The model under review builds one solid part; all positions refer to its coordinate system, in mm. A direction names the side the tool comes from. Give positions to 0.01 mm unless a question says otherwise; leave off trailing zeros. Loops run counter-clockwise (first coordinate to the right, second up) from the corner with the lowest first, then second, coordinate; pieces in that order, holes last. Notation, with made-up numbers: (1.25, -30.5) - (47.25, -30.5) arc R15 cw to (47.25, -11.5) - close; hole circle Ø3 at (-24, 44.25). An arc over 180 degrees is marked (long way). Answer as a JSON object with one key per item and string values.
from build123d import *

# Parameters (mm, degrees)
CROQUIS1_R              = 57
CROQUIS1_R_2            = 55.5
SALIENTE_EXTRUIR1_DEPTH = 530
CROQUIS2_R              = 10.65
CORTAR_EXTRUIR1_DEPTH   = 10
CROQUIS3_R              = 10.65
CORTAR_EXTRUIR3_DEPTH   = 10
CROQUIS4_W              = 120
CROQUIS4_H              = 120
CORTAR_EXTRUIR4_DEPTH   = 36
CORTAR_EXTRUIR5_DEPTH   = 36


with BuildPart() as part:
    # Croquis1 → Saliente-Extruir1 (new body)
    with BuildSketch(Plane(origin=(0, 0, 0), x_dir=(1, 0, 0), z_dir=(0, 1, 0))):
        with Locations(Location((0, 0, 0), (0, 0, 270))):
            Circle(CROQUIS1_R)
        with Locations(Location((0, 0, 0), (0, 0, 270))):
            Circle(CROQUIS1_R_2, mode=Mode.SUBTRACT)
    extrude(amount=SALIENTE_EXTRUIR1_DEPTH)

    # Croquis2 → Cortar-Extruir1 (cut)
    with BuildSketch(Plane.ZY.offset(57)):
        with Locations((0, 440)):
            Circle(CROQUIS2_R)
    extrude(amount=-CORTAR_EXTRUIR1_DEPTH, mode=Mode.SUBTRACT)

    # Croquis3 → Cortar-Extruir3 (cut)
    with BuildSketch(Plane(origin=(57, 0, 0), x_dir=(0, 0, -1), z_dir=(1, 0, 0))):
        with Locations((0, 38.1)):
            Circle(CROQUIS3_R)
    extrude(amount=-CORTAR_EXTRUIR3_DEPTH, mode=Mode.SUBTRACT)

    # Croquis4 → Cortar-Extruir4 (cut)
    with BuildSketch(Plane(origin=(40.305086528, 0, 40.305086528), x_dir=(0, -1, 0), z_dir=(0.7071067811865464, 0, 0.7071067811865488))):
        with Locations((-442.099170551, 0)):
            Rectangle(CROQUIS4_W, CROQUIS4_H)
    extrude(amount=-CORTAR_EXTRUIR4_DEPTH, mode=Mode.SUBTRACT)

    # Croquis6 → Cortar-Extruir5 (cut)
    with BuildSketch(Plane.ZY.offset(57)):
        with BuildLine():
            Line((4.146980327, 136.214628742), (-0.063914709, 136.214628742))
            add(Edge.make_bspline(
                [(-0.063914709, 136.214628742), (-0.467287481, 135.678507753), (-0.558467191, 135.016456308)],
                knots=[5.643669724, 5.643669724, 5.643669724, 6.14786855, 6.14786855, 6.14786855], degree=2, weights=[1, 0.968390884, 1]))
            add(Edge.make_bspline(
                [(-0.558467191, 135.016456308), (-0.963914609, 132.027107364), (2.041532809, 132.027107364), (5.046980227, 132.027107364), (4.641532809, 135.016456308)],
                knots=[4.577072223, 4.577072223, 4.577072223, 6.283185307, 6.283185307, 7.989298391, 7.989298391, 7.989298391], degree=2, weights=[1, 0.657683746, 1, 0.657683746, 1]))
            add(Edge.make_bspline(
                [(4.641532809, 135.016456308), (4.550353099, 135.678507753), (4.146980327, 136.214628742)],
                knots=[3.276909411, 3.276909411, 3.276909411, 3.781108237, 3.781108237, 3.781108237], degree=2, weights=[1, 0.968390884, 1]))
        make_face()
    extrude(amount=-CORTAR_EXTRUIR5_DEPTH, mode=Mode.SUBTRACT)


solid = part.part
Q1. Clearance check with flat-ended pins moving along their axes: pin 1 Ø1.5 at (y, z) = (124.5, -35) entering from +X; pin 2 Ø10 at (y, z) = (137.5, -42) entering from -X; pin 3 Ø6 at (x, y) = (17.5, 242) entering from -Z; pin 4 Ø1.3 at (x, z) = (-56, 1.5) entering from -Y. State where each tip first meets the part, or that it passes through.
Results:
{"pin 1": "stops at x = 45.56", "pin 2": "stops at x = -43.36", "pin 3": "stops at z = -55.12", "pin 4": "stops at y = 0"}
Q2. Consider section B-B, the plane z = -49. State the section outline as (x, y) points.
Results:
{"outline": "(-29.12, 0) - (-26.06, 0) - (-26.06, 530) - (-29.12, 530) - close; (26.06, 0) - (29.12, 0) - (29.12, 530) - (26.06, 530) - close"}
Q3. Consider section A-A, the plane x = 0. State the section outline as (y, z) points.
Results:
{"outline": "(0, -57) - (530, -57) - (530, -55.5) - (0, -55.5) - close; (0, 55.5) - (382.1, 55.5) - (382.1, 57) - (0, 57) - close; (502.1, 55.5) - (530, 55.5) - (530, 57) - (502.1, 57) - close"}
Q4. Consider section D-D, the plane y = 440. State the section outline as (x, z) points.
Results:
{"outline": "(-56, -10.65) arc R57 ccw to (52.32, -22.62) - (51.18, -21.48) arc R55.5 cw to (-54.47, -10.65) - close; (-56, 10.65) - (-54.47, 10.65) arc R55.5 cw to (-21.48, 51.18) - (-22.62, 52.32) arc R57 ccw to start"}
Q5. To check wall thickness, follow probe 1 along Y at (x, z) = (55.7, 0); probe 2 along Y at (x, z) = (-56, 0); probe 3 along Z at (x, y) = (-3, 497). State the ranges of each line that lie inside material, in increasing order. Write a range as [from, to].
Results:
{"probe 1": "y = [0, 27.45], [48.75, 382.1], [502.1, 530]", "probe 2": "y = [0, 133.01], [136.21, 429.35], [450.65, 530]", "probe 3": "z = [-56.92, -55.42]"}
Q6. The part is to be moulded in two halves that separate along Z. For faces 1 (the face through (-34.684, 261.29, -45.233)), 2 (the face through (40, 502.099, 40)), 3 (the face through (-55.75, 430.55, 4.91)), 4 (the face through (-33.771, 261.29, -44.043)), say which applies: +Z half, -Z half, draft (parallel to the pull), parting line (faces both ways), or undercut.
Results:
{"face 1": "parting line", "face 2": "draft", "face 3": "undercut", "face 4": "undercut"}
Q7. For faces 5 (the face through (40, 382.099, 40)), 6 (the face through (-55, 0, 12)), 7 (the face through (55.75, 28.65, -4.91)), list the 3-axis set-ups (+Z, -Z, +X, -X, +Y, -Y) from which the entire face can be reached by the end or side of a thin tool; tool diameter is ignored.
Results:
{"face 5": "+Z, +X", "face 6": "+Z, -Z, +X, -X, -Y", "face 7": "+X"}
Q8. Consider section C-C, the plane z = 25. State the section outline as (x, y) points (3 decimals).
Results:
{"outline": "(-51.225, 0) - (-49.55, 0) - (-49.55, 530) - (-51.225, 530) - close; (49.55, 0) - (51.225, 0) - (51.225, 382.099) - (49.55, 382.099) - close; (49.55, 502.099) - (51.225, 502.099) - (51.225, 530) - (49.55, 530) - close"}
